```python
from build123d import *

# Parameters (mm, degrees)
SKETCH1_W           = 48
SKETCH1_H           = 16
SKETCH1_R           = 1.85
BOSS_EXTRUDE1_DEPTH = 4
BOSS_EXTRUDE2_DEPTH = 16
FILLET1_R           = 4
FILLET2_R           = 8


with BuildPart() as part:
    # Sketch1 → Boss-Extrude1 (new body)
    with BuildSketch(Plane(origin=(0, 0, 0), x_dir=(1, 0, 0), z_dir=(0, 1, 0))):
        Rectangle(SKETCH1_W, SKETCH1_H)
        with Locations(Location((-16, 0, 0), (0, 0, 270))):
            Circle(SKETCH1_R, mode=Mode.SUBTRACT)
        with Locations(Location((16, 0, 0), (0, 0, 270))):
            Circle(SKETCH1_R, mode=Mode.SUBTRACT)
    extrude(amount=BOSS_EXTRUDE1_DEPTH)

    # Sketch2 → Boss-Extrude2 (add)
    with BuildSketch(Plane.ZY.offset(8)):
        Polygon((-8, 4), (-8, 0), (-12, 0), (-12, 11.5), (12, 11.5), (12, 0), (8, 0), (8, 4), (8, 7.5), (-8, 7.5), align=None)
    extrude(amount=-BOSS_EXTRUDE2_DEPTH)

    # Fillet1
    fillet1_edges = [part.edges().sort_by_distance(p)[0] for p in [
        (0, 11.5, 12),
        (0, 0, 12),
        (0, 0, -12),
        (0, 11.5, -12),
    ]]
    fillet(fillet1_edges, radius=FILLET1_R)

    # Fillet2
    fillet2_edges = [part.edges().sort_by_distance(p)[0] for p in [
        (-24, 2, 8),
        (-24, 2, -8),
        (24, 2, 8),
        (24, 2, -8),
    ]]
    fillet(fillet2_edges, radius=FILLET2_R - 0.0001)  # a hair under: the kernel refuses the full size


solid = part.part
```
Geometry: final body of the model. Coordinates: model frame, mm. A direction names the side the tool comes from. Give positions to 0.01 mm unless a question says otherwise; leave off trailing zeros. Loops run counter-clockwise (first coordinate to the right, second up) from the corner with the lowest first, then second, coordinate; pieces in that order, holes last. Notation, with made-up numbers: (-39.5, 44) - (3.5, 44) arc R11 ccw to (3.5, 50) - close; hole circle Ø6 at (37, -24.5). An arc over 180 degrees is marked (long way). Answer as CSV lines item,"result". Start each with the question number.
(1) Section query B-B (z = -1.25). Output: boundary loops of the cut face in (x, y), and give its area (3 significant figures).
(2) Pin query (flat end, axial travel): P1, Ø2, axis at x = -13, y = 2.5, coming from the +Z side; P2, Ø3, axis at x = 5.5, y = 1, coming from the +Z side; P3, Ø1, axis at x = -18, z = 2.5, coming from the +Y side; P4, Ø2, axis at x = -16, z = 0, coming from the -Y side. Return the tip coordinate at first contact, or that it passes through.
(3) Section query D-D (y = 10). Output: boundary loops of the cut face in (x, z), and give its area (3 significant figures).
(4) Section query A-A (x = -6.5). Output: boundary loops of the cut face in (y, z), and give its area (3 significant figures).
(5) Reachability of faces 4 (the face through (12, 2, -8)), 5 (the face through (12, 2, 8)), 6 (the face through (-12, 2, -8)), 7 (the face through (-12, 2, 8)), 8 (the face through (0, 6, 8)) from +Z, -Z, +X, -X, +Y, -Y: full face, straight path, thin tool, end or side. Return the list, or none.
(6) Ray query, line 1 along X through (y, z) = (1.9, 0); line 2 along Y through (x, z) = (-0.5, -4.25); line 3 along Z through (x, y) = (2, 6). Return the intervals inside material, ascending. Write a range as [from, to].
(7) Mould query, pull axis Y, two halves, no side actions, for faces 1 (the face through (0, 6, -8)), 2 (the face through (0.112, 1.141, 10.797)), 3 (the face through (17.834, 1.972, -0.241)). Classes: +Y half, -Y half, draft (parallel to the pull), parting line (faces both ways), or undercut.
(8) Section query C-C (z = 4.5). Output: boundary loops of the cut face in (x, y), and give its area (3 significant figures).
Worked answers:
1,outline,"(-23.9, 0) - (-17.36, 0) - (-17.36, 4) - (-23.9, 4) - close; (-14.64, 0) - (14.64, 0) - (14.64, 4) - (-14.64, 4) - close; (-8, 7.5) - (8, 7.5) - (8, 11.5) - (-8, 11.5) - close; (17.36, 0) - (23.9, 0) - (23.9, 4) - (17.36, 4) - close"
1,area,"233 mm^2"
2,P1,"stops at z = 8"
2,P2,"stops at z = 11.71"
2,P3,"stops at y = 4"
2,P4,"passes through"
3,outline,"(-8, -11.12) - (8, -11.12) - (8, 11.12) - (-8, 11.12) - close"
3,area,"356 mm^2"
4,outline,"(0, -8) arc R4 ccw to (4, -12) - (7.5, -12) arc R4 ccw to (11.5, -8) - (11.5, 8) arc R4 ccw to (7.5, 12) - (4, 12) arc R4 ccw to (0, 8) - close; hole (4, -8) - (7.5, -8) - (7.5, 8) - (4, 8) - close"
4,area,"206 mm^2"
5,face 4,"-Z, +X, +Y, -Y"
5,face 5,"+Z, +X, +Y, -Y"
5,face 6,"-Z, -X, +Y, -Y"
5,face 7,"+Z, -X, +Y, -Y"
5,face 8,"+X, -X"
6,line 1,"x = [-24, -17.85], [-14.15, 14.15], [17.85, 24]"
6,line 2,"y = [0, 4], [7.5, 11.5]"
6,line 3,"z = [-12, -8], [8, 12]"
7,face 1,"undercut"
7,face 2,"-Y half"
7,face 3,"draft"
8,outline,"(-22.61, 0) - (22.61, 0) - (22.61, 4) - (-22.61, 4) - close; (-8, 7.5) - (8, 7.5) - (8, 11.5) - (-8, 11.5) - close"
8,area,"245 mm^2"
